from build123d import *

# Parameters (mm, degrees)
SKETCH1_W           = 52.200247598
SKETCH1_H           = 6.332152384
BOSS_EXTRUDE1_DEPTH = 2.5
FILLET1_R           = 2
FILLET2_R           = 2
SKETCH4_W           = 48.201423078
SKETCH4_H           = 8.78902621
BOSS_EXTRUDE2_DEPTH = 1.8
FILLET3_R           = 2
FILLET4_R           = 2


with BuildPart() as part:
    # Sketch1 → Boss-Extrude1 (new body)
    with BuildSketch(Plane(origin=(0, -35, 0), x_dir=(1, 0, 0), z_dir=(0, 1, 0))):
        with Locations((60.097811714, 35.152469917)):
            Rectangle(SKETCH1_W, SKETCH1_H)
    extrude(amount=-BOSS_EXTRUDE1_DEPTH)

    # Fillet1
    fillet1_edges = [part.edges().sort_by_distance(p)[0] for p in [
        (60.097811714, -37.5, -38.318546109),
    ]]
    fillet(fillet1_edges, radius=FILLET1_R)

    # Fillet2
    fillet2_edges = [part.edges().sort_by_distance(p)[0] for p in [
        (86.197935513, -37.5, -34.152469917),
        (86.197935513, -35.25, -38.318546109),
        (33.997687915, -35.25, -38.318546109),
        (33.997687915, -37.5, -34.152469917),
        (33.997687915, -36.914213562, -37.732759671),
        (86.197935513, -36.914213562, -37.732759671),
    ]]
    fillet(fillet2_edges, radius=FILLET2_R)


with BuildPart() as boss_extrude2_tool:
    # Sketch4 → Boss-Extrude2 (new body)
    with BuildSketch(Plane.XZ.offset(37.5)):
        with Locations((60.098399454, -31.924033004)):
            Rectangle(SKETCH4_W, SKETCH4_H)
    extrude(amount=BOSS_EXTRUDE2_DEPTH)


with BuildPart() as part_1:
    add(part.part)


with BuildPart() as part_2:
    # Boss-Extrude2: joined with boss_extrude2_tool
    add(part_1.part.fuse(boss_extrude2_tool.part, tol=0.00001))

    # Fillet3
    # the kernel refuses this fillet: 2 mm, written as the material it takes off along each edge
    with BuildSketch(Plane(origin=(89.174048179, -39.3, -27.529519899), x_dir=(0, 0, -1), z_dir=(-1, 0, 0))) as fillet3_piece_1:
        with BuildLine():
            CenterArc((1.989974874, -2), FILLET3_R, 90, 84.260829523)
            Line((0, -1.8), (-0.039799497, -1.796))
            ThreePointArc((-0.039799497, -1.796), (-0.04, -0.9), (-0.04, 0))
            Line((-0.04, 0), (0, 0.04))
            Line((0, 0.04), (1.989974874, 0.04))
            Line((1.989974874, 0.04), (1.989974874, 0))
        make_face()
    extrude(amount=58.151297449, mode=Mode.SUBTRACT)

    # Fillet4
    # the kernel refuses this fillet: 2 mm, written as the material it takes off along each edge
    with BuildSketch(Plane(origin=(31.02275073, -39.3, -36.318546109), x_dir=(0, 1, 0), z_dir=(1, 0, 0))) as fillet4_piece_1:
        with BuildLine():
            CenterArc((2, 1.989974874), FILLET4_R, 180, 84.260829523)
            Line((0, 1.989974874), (-0.04, 1.989974874))
            Line((-0.04, 1.989974874), (-0.04, 0))
            Line((-0.04, 0), (0, -0.04))
            ThreePointArc((0, -0.04), (0.9, -0.04), (1.796, -0.039799497))
            Line((1.796, -0.039799497), (1.8, 0))
        make_face()
    extrude(amount=58.151297449, mode=Mode.SUBTRACT)


solid = part_2.part
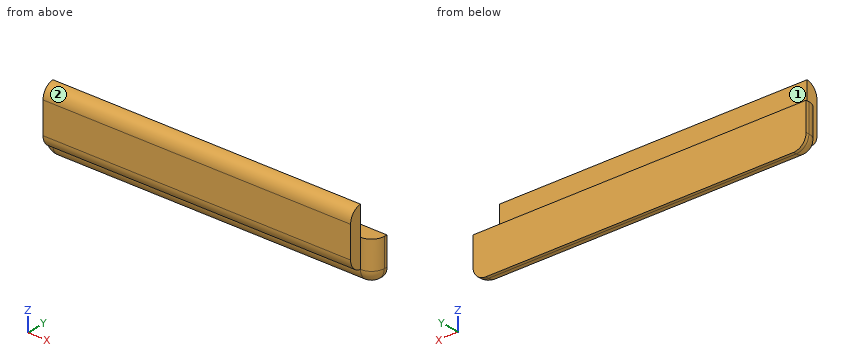
Part model, mm, in its own coordinate system. Face numbers are marked on the shaded views. A direction names the side the tool comes from. Coordinates: 2 decimals unless noted, no trailing zeros. Write each loop counter-clockwise with the first axis right and the second up, starting at its lowest first coordinate (ties: lowest second). Pieces come first, ordered by that corner, then holes. Notation, with made-up numbers: (64.25, 58.25) - (84.25, 58.25) arc R23 cw to (84.25, 69.25) - close; hole circle Ø7 at (-30.5, 62). An arc over 180 degrees is marked (long way). Put each result on its own line as item: value.
1. Probe line 1 along Z through (x, y) = (48.5, -35.7); line 2 along Y through (x, z) = (79.5, -30.5); line 3 along Y through (x, z) = (41.5, -34.5). List the from-to ranges inside material, lowest first. Write a range as [from, to].
Final values:
line 1: z = [-38.31, -31.99]
line 2: y = [-39.3, -37.5]
line 3: y = [-39.29, -35]
2. 3-axis set-ups, long thin cutter, end or side, ignore diameter. For the marked faces 1 and 2: which of +Z, -Z, +X, -X, +Y, -Y reach the whole face in a straight line?
Final values:
face 1: +Z, +X, -X, +Y
face 2: +Z, +X, -X, -Y
3. Band-saw the part on D-D (z = -30). Write the cut outline in (x, y).
Final values:
outline: (36, -39.3) - (84.2, -39.3) - (84.2, -37.5) - (36, -37.5) - close
4. Band-saw the part on A-A (z = -33). Write the cut outline in (x, y).
Final values:
outline: (34, -35.5) arc R2 ccw to (36, -37.5) - (36, -39.3) - (84.2, -39.3) - (84.2, -37.5) arc R2 ccw to (86.2, -35.5) - (86.2, -35) - (34, -35) - close
5. Band-saw the part on C-C (y = -36.3). Write the cut outline in (x, z), then the cut area to 3 significant figures.
Final values:
outline: (34.16, -36.32) arc R1.83 ccw to (36, -38.15) - (84.2, -38.15) arc R1.83 ccw to (86.03, -36.32) - (86.03, -31.99) - (34.16, -31.99) - close
area: 318 mm²
6. Band-saw the part on B-B (x = 47.5). Write the cut outline in (y, z), then the cut area to 3 significant figures.
Final values:
outline: (-39.3, -34.33) arc R2 ccw to (-37.5, -36.32) arc R2 ccw to (-35.5, -38.32) - (-35, -38.32) - (-35, -31.99) - (-37.5, -31.99) - (-37.5, -27.53) arc R2 ccw to (-39.3, -29.52) - close
area: 29.1 mm²
7. Flat gauge pins, fed straight in: pin 1 Ø0.9 at (y, z) = (-38.5, -32.5) entering from -X; pin 2 Ø1 at (x, y) = (59.5, -36) entering from +Z; pin 3 Ø1 at (x, y) = (62.5, -39) entering from +Z. Where does each tip first touch, or does it go through?
Final values:
pin 1: stops at x = 36
pin 2: stops at z = -31.99
pin 3: stops at z = -27.92
